Build history of the part. All positions in model axes, mm. Face numbers are marked on the shaded views. Give positions to 0.01 mm unless a question says otherwise; leave off trailing zeros. Order: outer loops, then holes, each group sorted by start corner. A loop starts at its lowest first (then second) coordinate and runs counter-clockwise, first axis right, second up. Notation, with made-up numbers: M 42.5,-39.75 L 99.5,-39.75 A21 cw 99.5,-13.75 Z; hole C -3.5,50 d6. An arc over 180 degrees is marked long. Use CSV: the item, a comma, the result in double quotes. Start each with the question number.
Item 1: Wall check: line 1 along Z through (x, y) = (2.75, -0.75); line 2 along X through (y, z) = (-0.2, 1.5); line 3 along X through (y, z) = (-0.9, 2.5). Give the ranges that are in metal, low to high.
Item 2: Band-saw the part on A-A on z = 1.7. Write the cut outline in (x, y).
Item 3: Band-saw the part on B-B on x = 2.8. Write the cut outline in (y, z), plus the area to 3 significant figures.
Item 4: Band-saw the part on C-C on y = -0.35. Write the cut outline in (x, z).
Item 5: Two-plate mould, pull along X, no slides. Class the marked faces 1, 2 and 3: pulls with the +X half, pulls with the -X half, needs draft (parallel to the pull), parting line crosses it, or undercut.
from build123d import *

# Parameters (mm, degrees)
F0_W     = 20
F0_H     = 8.6
F1_DEPTH = 1.5
F2_R     = 1.1
F3_DEPTH = 1.5
F4_R     = 1


with BuildPart() as f1:
    # F0 (on Front) → F1 (new body)
    with BuildSketch(Plane.XZ):
        with Locations((10, 4.3)):
            Rectangle(F0_W, F0_H)
    extrude(amount=F1_DEPTH)

    # F2 (on face) → F3 (cut, through all)
    with BuildSketch(Plane.XZ.offset(1.5)):
        with Locations((2.8, 6.9)):
            Circle(F2_R)
        with Locations((17.2, 6.9)):
            Circle(F2_R)
        with Locations((2.8, 1.7)):
            Circle(F2_R)
        with Locations((17.2, 1.7)):
            Circle(F2_R)
    extrude(amount=-F3_DEPTH, mode=Mode.SUBTRACT)

    # F4
    f4_edges = [f1.edges().sort_by_distance(p)[0] for p in [
        (20, -0.75, 8.6),
        (20, -0.75, 0),
        (0, -0.75, 8.6),
        (0, -0.75, 0),
    ]]
    fillet(f4_edges, radius=F4_R)


solid = f1.part
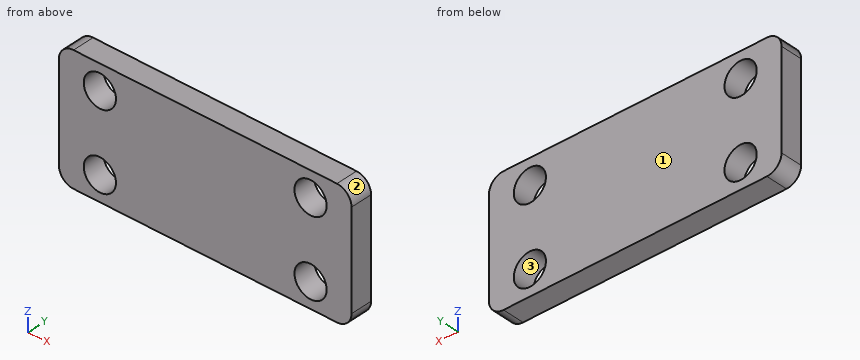
Model answer:
1,line 1,"z = 0 to 0.6, 2.8 to 5.8, 8 to 8.6"
1,line 2,"x = 0 to 1.72, 3.88 to 16.12, 18.28 to 20"
1,line 3,"x = 0 to 2.05, 3.55 to 16.45, 17.95 to 20"
2,outline,"M 0,-1.5 L 1.7,-1.5 L 1.7,0 L 0,0 Z; M 3.9,-1.5 L 16.1,-1.5 L 16.1,0 L 3.9,0 Z; M 18.3,-1.5 L 20,-1.5 L 20,0 L 18.3,0 Z"
3,outline,"M -1.5,0 L 0,0 L 0,0.6 L -1.5,0.6 Z; M -1.5,2.8 L 0,2.8 L 0,5.8 L -1.5,5.8 Z; M -1.5,8 L 0,8 L 0,8.6 L -1.5,8.6 Z"
3,area,"6.30 mm^2"
4,outline,"M 0,1 A1 ccw 1,0 L 19,0 A1 ccw 20,1 L 20,7.6 A1 ccw 19,8.6 L 1,8.6 A1 ccw 0,7.6 Z; hole C 2.8,1.7 d2.2; hole C 2.8,6.9 d2.2; hole C 17.2,1.7 d2.2; hole C 17.2,6.9 d2.2"
5,face 1,"needs draft"
5,face 2,"pulls with the +X half"
5,face 3,"undercut"
